```python
from build123d import *

# Parameters (mm, degrees)
SKETCH1_R                = 92.075
SKETCH1_R_2              = 79.375
BOSS_EXTRUDE1_DEPTH      = 69.85
SKETCH2_R                = 92.075
BOSS_EXTRUDE2_DEPTH      = 12.7
SKETCH3_R                = 8.73125
CUT_EXTRUDE1_DEPTH       = 12.7
SKETCH4_R                = 2.38125
CUT_EXTRUDE2_DEPTH       = 19.05
BOSS_EXTRUDE3_START      = -12.7
BOSS_EXTRUDE3_DEPTH      = 12.7
SKETCH7_W                = 127
SKETCH7_H                = 38.1
CUT_EXTRUDE4_DEPTH       = 139.7
SKETCH8_W                = 127
SKETCH8_H                = 6.35
BOSS_EXTRUDE4_DEPTH      = 139.7
BOSS_EXTRUDE5_DEPTH      = 139.7
BOSS_EXTRUDE6_START      = -6.35
BOSS_EXTRUDE6_DEPTH      = 6.35
BOSS_EXTRUDE7_DEPTH      = 6.35
REVOLVE1_ANGLE           = 21
REVOLVE1_OTHER_WAY_ANGLE = 21
SKETCH14_R               = 2.778125
CUT_EXTRUDE5_DEPTH       = 9.525


with BuildPart() as part:
    # Sketch1 → Boss-Extrude1 (new, symmetric)
    with BuildSketch(Plane(origin=(0, 0, 0), x_dir=(1, 0, 0), z_dir=(0, 1, 0))):
        with Locations(Location((0, 0, 0), (0, 0, 270))):
            Circle(SKETCH1_R)
        with Locations(Location((0, 0, 0), (0, 0, 270))):
            Circle(SKETCH1_R_2, mode=Mode.SUBTRACT)
    extrude(amount=BOSS_EXTRUDE1_DEPTH, both=True)

    # Sketch2 → Boss-Extrude2 (add)
    with BuildSketch(Plane.XZ.offset(69.85)):
        with Locations(Location((0, 0, 0), (0, 0, 270))):
            Circle(SKETCH2_R)
    extrude(amount=BOSS_EXTRUDE2_DEPTH)

    # Sketch3 → Cut-Extrude1 (cut)
    with BuildSketch(Plane.XZ.offset(82.55)):
        with Locations(Location((0, 0, 0), (0, 0, 270))):
            Circle(SKETCH3_R)
    extrude(amount=-CUT_EXTRUDE1_DEPTH, mode=Mode.SUBTRACT)

    # Sketch4 → Cut-Extrude2 (cut)
    with BuildSketch(Plane(origin=(0, 69.85, 0), x_dir=(1, 0, 0), z_dir=(0, 1, 0))):
        with Locations(Location((0, 85.09, 0), (0, 0, 270))):
            Circle(SKETCH4_R)
        with Locations(Location((73.690101608, -42.545, 0), (0, 0, 270))):
            Circle(SKETCH4_R)
        with Locations(Location((-73.690101608, -42.545, 0), (0, 0, 270))):
            Circle(SKETCH4_R)
    extrude(amount=-CUT_EXTRUDE2_DEPTH, mode=Mode.SUBTRACT)

    # Sketch6 → Boss-Extrude3 (add)
    with BuildSketch(Plane.XZ.offset(82.55).offset(BOSS_EXTRUDE3_START)):
        with BuildLine():
            Line((127, 92.075), (0, 92.075))
            ThreePointArc((0, 92.075), (41.881126418, 81.99863947), (74.59560979, 53.975))
            Line((74.59560979, 53.975), (127, 53.975))
            Line((127, 53.975), (127, 92.075))
        make_face()
    extrude(amount=BOSS_EXTRUDE3_DEPTH)

    # Sketch7 → Cut-Extrude4 (cut)
    with BuildSketch(Plane(origin=(0, 69.85, 0), x_dir=(1, 0, 0), z_dir=(0, 1, 0))):
        with Locations((63.5, -73.025)):
            Rectangle(SKETCH7_W, SKETCH7_H)
    extrude(amount=-CUT_EXTRUDE4_DEPTH, mode=Mode.SUBTRACT)

    # Sketch8 → Boss-Extrude4 (add)
    with BuildSketch(Plane(origin=(0, -69.85, 0), x_dir=(1, 0, 0), z_dir=(0, 1, 0))):
        with Locations((63.5, -88.9)):
            Rectangle(SKETCH8_W, SKETCH8_H)
    extrude(amount=BOSS_EXTRUDE4_DEPTH)

    # Sketch9 → Boss-Extrude5 (add)
    with BuildSketch(Plane(origin=(0, -69.85, 0), x_dir=(1, 0, 0), z_dir=(0, 1, 0))):
        with BuildLine():
            Line((127, -53.975), (58.198711326, -53.975))
            ThreePointArc((58.198711326, -53.975), (54.984921313, -57.245515573), (51.587643869, -60.325))
            Line((51.587643869, -60.325), (127, -60.325))
            Line((127, -60.325), (127, -53.975))
        make_face()
    extrude(amount=BOSS_EXTRUDE5_DEPTH)

    # Sketch10 → Boss-Extrude6 (add)
    with BuildSketch(Plane(origin=(0, 69.85, 0), x_dir=(1, 0, 0), z_dir=(0, 1, 0)).offset(BOSS_EXTRUDE6_START)):
        with BuildLine():
            ThreePointArc((0, -79.375), (27.49630657, -74.460350187), (51.587643869, -60.325))
            Line((51.587643869, -60.325), (127, -60.325))
            Line((127, -60.325), (127, -85.725))
            Line((127, -85.725), (0, -85.725))
            Line((0, -85.725), (0, -79.375))
        make_face()
    extrude(amount=BOSS_EXTRUDE6_DEPTH)

    # Sketch11 → Boss-Extrude7 (add)
    with BuildSketch(Plane(origin=(0, 69.85, 0), x_dir=(1, 0, 0), z_dir=(0, 1, 0))):
        with BuildLine():
            ThreePointArc((-83.822405269, -38.1), (-92.075, 0), (-83.822405269, 38.1))
            Line((-83.822405269, 38.1), (-130.175, 38.1))
            Line((-130.175, 38.1), (-130.175, -38.1))
            Line((-130.175, -38.1), (-83.822405269, -38.1))
        make_face()
        with BuildLine():
            Line((83.822405269, -38.1), (130.175, -38.1))
            Line((130.175, -38.1), (130.175, 38.1))
            Line((130.175, 38.1), (83.822405269, 38.1))
            ThreePointArc((83.822405269, 38.1), (92.075, 0), (83.822405269, -38.1))
        make_face()
    extrude(amount=-BOSS_EXTRUDE7_DEPTH)

    # Sketch13 → Revolve1 (revolve)
    with BuildSketch(Plane.XY):
        Polygon((92.075, 63.5), (92.075, 47.625), (104.775, 63.5), align=None)
        Polygon((-92.075, 63.5), (-92.075, 47.625), (-104.775, 63.5), align=None)
    revolve(axis=Axis((0, -102.398385613, 0), (0, 1, 0)), revolution_arc=REVOLVE1_ANGLE)

    # Sketch13 → Revolve1 other way (revolve)
    with BuildSketch(Plane.XY):
        Polygon((92.075, 63.5), (92.075, 47.625), (104.775, 63.5), align=None)
        Polygon((-92.075, 63.5), (-92.075, 47.625), (-104.775, 63.5), align=None)
    revolve(axis=Axis((0, -102.398385613, 0), (0, -1, 0)), revolution_arc=REVOLVE1_OTHER_WAY_ANGLE)

    # Sketch14 → Cut-Extrude5 (cut)
    with BuildSketch(Plane(origin=(0, 69.85, 0), x_dir=(1, 0, 0), z_dir=(0, 1, 0))):
        with Locations(Location((-117.475, 0, 0), (0, 0, 180))):
            Circle(SKETCH14_R)
        with Locations(Location((117.475, 0, 0), (0, 0, 180))):
            Circle(SKETCH14_R)
    extrude(amount=-CUT_EXTRUDE5_DEPTH, mode=Mode.SUBTRACT)


solid = part.part
```
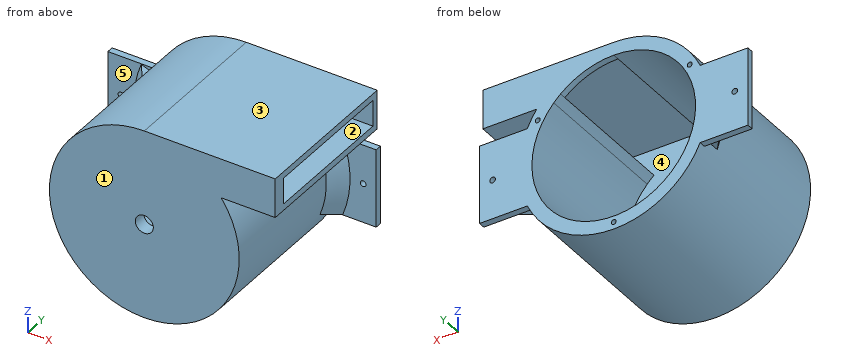
Verification items for the finished model (mm, model axes). Face numbers are marked on the shaded views. A direction names the side the tool comes from. Coordinates: 2 decimals unless noted, no trailing zeros. Loops run counter-clockwise (first coordinate to the right, second up) from the corner with the lowest first, then second, coordinate; pieces in that order, holes last. Notation, with made-up numbers: (37, 84.25) - (91, 84.25) arc R17 ccw to (91, 99.25) - close; hole circle Ø2 at (45, -8.75). An arc over 180 degrees is marked (long way). Return JSON: item names as keys, results as strings.
1. Thickness scan on L1, parallel to X at y = 3, z = 2; L2, parallel to Y at x = 105.5, z = 67.5; L3, parallel to X at y = 35, z = 23.5. Record the ranges inside material, lowest first.
Established:
{"L1": "x = -92.05 to -79.35, 79.35 to 92.05", "L2": "y = -82.55 to -69.85, 63.5 to 69.85", "L3": "x = -89.03 to -75.82, 75.82 to 89.03"}
2. Tool access check on the marked faces 1 and 2. Record the directions out of +Z, -Z, +X, -X, +Y, -Y that give a thin tool (end or side, any length) a straight path to the whole face; none if there is none.
Established:
{"face 1": "+Z, -Z, +X, -X, -Y", "face 2": "+X"}
3. Section check C-C, the plane z = -54. Record the boundary of the cut face in (x, y), then the cut area to 3 significant figures.
Established:
{"outline": "(-74.58, -82.55) - (74.58, -82.55) - (74.58, 69.85) - (58.18, 69.85) - (58.18, -69.85) - (-58.18, -69.85) - (-58.18, 69.85) - (-74.58, 69.85) - close", "area": "6,480 mm2"}
4. Section check A-A, the plane y = -43. Record the boundary of the cut face in (x, z) (3 decimals), then the cut area to 3 significant figures.
Established:
{"outline": "(0, 79.375) - (0, 85.725) - (127, 85.725) - (127, 92.075) - (0, 92.075) arc R92.075 ccw (long way) to (74.596, 53.975) - (127, 53.975) - (127, 60.325) - (51.588, 60.325) arc R79.375 cw (long way) to start", "area": "7,140 mm2"}
5. Mould release check, pull along Z, two halves, no side actions. Record for the marked faces 3, 4 and 5: +Z half, -Z half, draft (parallel to the pull), parting line (faces both ways), or undercut.
Established:
{"face 3": "+Z half", "face 4": "undercut", "face 5": "draft"}
6. Section check B-B, the plane x = 35.5. Record the boundary of the cut face in (y, z) (3 decimals), then the cut area to 3 significant figures.
Established:
{"outline": "(-82.55, -84.956) - (69.85, -84.956) - (69.85, -70.994) - (-69.85, -70.994) - (-69.85, 85.725) - (63.5, 85.725) - (63.5, 70.994) - (69.85, 70.994) - (69.85, 92.075) - (-82.55, 92.075) - close", "area": "5,180 mm2"}
7. Section check D-D, the plane x = -41. Record the boundary of the cut face in (y, z).
Established:
{"outline": "(-82.55, -82.44) - (69.85, -82.44) - (69.85, -67.97) - (-69.85, -67.97) - (-69.85, 67.97) - (69.85, 67.97) - (69.85, 82.44) - (-82.55, 82.44) - close"}
8. Go/stop test with flat-tipped pins: pin 1 (3.5 mm diameter, centred on x = 117.475, z = 0, fed in from -Y); pin 2 (2.5 mm diameter, centred on x = -1, z = -85.5, fed in from +Y); pin 3 (5 mm diameter, centred on y = 15.5, z = 81, fed in from +X); pin 4 (3 mm diameter, centred on y = 49, z = 48.5, fed in from -X). Record where each tip stops, or that it passes through.
Established:
{"pin 1": "passes through", "pin 2": "stops at y = 50.8", "pin 3": "stops at x = 0", "pin 4": "stops at x = -79.18"}
